Answer from the drawing. Dimensions are ordinates in mm from the lowest x, y and z of the part. A direction names the side the tool comes from. Coordinates: 2 decimals unless noted, no trailing zeros. Write each loop counter-clockwise with the first axis right and the second up, starting at its lowest first coordinate (ties: lowest second). Pieces come first, ordered by that corner, then holes. Notation, with made-up numbers: (84.25, 66) - (111.25, 66) arc R15 cw to (111.25, 82) - close; hole circle Ø7 at (73.25, 35). An arc over 180 degrees is marked (long way). Answer as a JSON object with one key per item and string values. Group by question number.
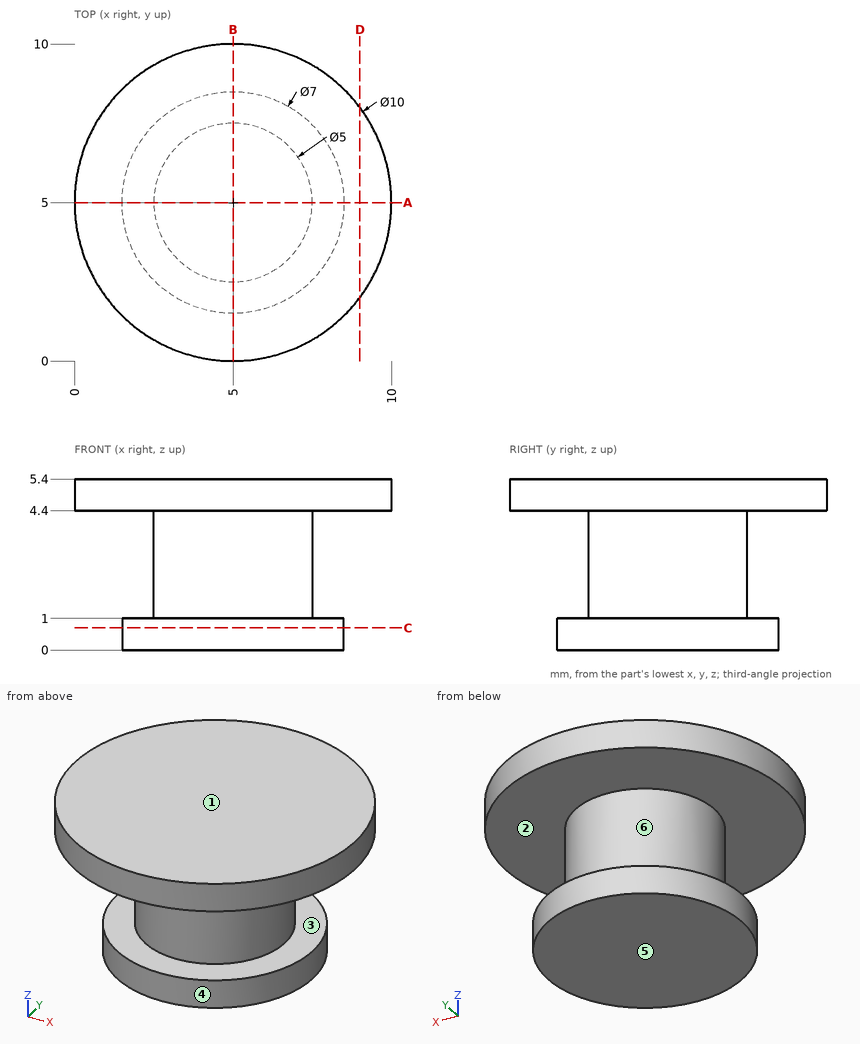
Q1. Section C-C on z = 0.7 is taken. Determine the outline of the cut face in (x, y), plus the area to 3 significant figures.
Q2. Section D-D on x = 9 is taken. Determine the outline of the cut face in (y, z), plus the area to 3 significant figures.
Q3. For a pull along Z with two mould halves and no side action, classify the marked faces 3, 4, 5 and 6 as +Z half, -Z half, draft (parallel to the pull), parting line (faces both ways), or undercut.
Q4. Consider L1, parallel to Z at x = 8, y = 5.25; L2, parallel to Z at x = 1.25, y = 4; L3, parallel to Y at x = 3.75, z = 3.9. Determine where each line is inside the solid, lowest interval first. Write a range as from..to.
Q5. A tool of negligible diameter and unlimited length cuts with its end or side. For the marked faces 1 and 2, from which of +Z, -Z, +X, -X, +Y, -Y can it reach the whole face along a straight path? Write none if from no direction.
Q6. Flat-ended cylindrical pins translate along their axes: pin 1 Ø1.5 at (y, z) = (2.5, 3) entering from +X; pin 2 Ø1 at (y, z) = (6.5, 1) entering from -X; pin 3 Ø1.5 at (y, z) = (2.5, 3) entering from -X. Find the tip coordinate at first contact, or state that the pin passes through.
Q7. Section A-A on y = 5 is taken. Determine the outline of the cut face in (x, z).
Numbers:
{
 "1": {"outline": "circle Ø7 at (5, 5)", "area": "38.5 mm²"},
 "2": {"outline": "(2, 4.4) - (8, 4.4) - (8, 5.4) - (2, 5.4) - close", "area": "6.00 mm²"},
 "3": {"face 3": "undercut", "face 4": "draft", "face 5": "-Z half", "face 6": "undercut"},
 "4": {"L1": "z = 0..1, 4.4..5.4", "L2": "z = 4.4..5.4", "L3": "y = 2.83..7.17"},
 "5": {"face 1": "+Z, +X, -X, +Y, -Y", "face 2": "none"},
 "6": {"pin 1": "stops at x = 6.79", "pin 2": "stops at x = 1.65", "pin 3": "stops at x = 3.21"},
 "7": {"outline": "(0, 4.4) - (2.5, 4.4) - (2.5, 1) - (1.5, 1) - (1.5, 0) - (8.5, 0) - (8.5, 1) - (7.5, 1) - (7.5, 4.4) - (10, 4.4) - (10, 5.4) - (0, 5.4) - close"}
}
